Autodesk Fusion 360 part; units mm, degrees
sketch "Sketch1" plane through (0, 0, 0) normal (0, 1, 0) x (1, 0, 0)
  line L0 (13, 29) -> (-13, 29) construction
  line L1 (-13, 29) -> (-13, -29) construction
  line L2 (-13, -29) -> (13, -29) construction
  line L3 (13, -29) -> (13, 29) construction
  line L4 (13, 29) -> (-13, -29) construction
  line L5 (-13, 29) -> (13, -29) construction
  line L6 (0, 0) -> (0, 16.0365) construction
  line L7 (0, 0) -> (-11.1519, 0) construction
  line L8 (20, 36) -> (-20, 36)
  line L9 (-20, 36) -> (-20, -36)
  line L10 (-20, -36) -> (20, -36)
  line L11 (20, -36) -> (20, 36)
  line L12 (20, 36) -> (-20, -36) construction
  line L13 (-20, 36) -> (20, -36) construction
  circle A0 centre (13, 29) radius 1.75
  circle A1 centre (-13, 29) radius 1.75
  circle A2 centre (13, -29) radius 1.75
  circle A3 centre (-13, -29) radius 1.75
  line L14 (7.5, 36) -> (-7.5, 36)
  line L15 (-7.5, 36) -> (-7.5, 56)
  line L16 (-7.5, 56) -> (7.5, 56)
  line L17 (7.5, 56) -> (7.5, 36)
  line L18 (7.5, 36) -> (-7.5, 56) construction
  line L19 (-7.5, 36) -> (7.5, 56) construction
  circle A4 centre (0, 48) radius 3.4
  line L20 (7.5, -56) -> (7.5, -36)
  line L21 (-7.5, -56) -> (7.5, -56)
  line L22 (-7.5, -36) -> (-7.5, -56)
  circle A5 centre (0, -48) radius 3.4
  line L23 (7.5, -36) -> (-7.5, -36)
  point P0 (0, 46)
  dimension "d1" = 3.5
  dimension "d2" = 58
  dimension "d3" = 26
  dimension "d4" = 7
  dimension "d5" = 7
  dimension "d6" = 15
  dimension "d7" = 20
  dimension "d8" = 6.8
  dimension "d9" = 12
extrude "Extrude1" add sketch "Sketch1" along normal blind 4
fillet "Fillet1" radius 3 12 edges at (7.5, 2, 36) (20, 2, 36) (7.5, 2, 56) (-7.5, 2, 56) (-20, 2, 36) (-7.5, 2, 36) (20, 2, -36) (7.5, 2, -36) (7.5, 2, -56) (-7.5, 2, -56) (-20, 2, -36) (-7.5, 2, -36)
chamfer "Chamfer1" distance 2 angle 45 4 edges at (-14.6316, 4, -29.6328) (11.3684, 4, -29.6328) (11.3684, 4, 28.3672) (-14.6316, 4, 28.3672)
Can you work these out from the model? Positions are in its coordinate system, mm. A direction names the side the tool comes from. Coordinates: 2 decimals unless noted, no trailing zeros. Loops run counter-clockwise (first coordinate to the right, second up) from the corner with the lowest first, then second, coordinate; pieces in that order, holes last. Notation, with made-up numbers: M -29,89 L -17,89 A23 cw -17,116 Z; hole C 55,29 d1. An arc over 180 degrees is marked long. Return JSON: item names as keys, results as strings. Group by question number.
Item 1: If I drill on L1, parallel to X at y = 1.1, z = 29; L2, parallel to Z at x = -13, y = 2; L3, parallel to Z at x = 0, y = 2.8, over which ranges is the centre line in solid material (lowest first)? Write a range as from..to.
Item 2: Thinking about a two-plate mould opening in Z: for faces 1 (the cylindrical face through (-6.6, 2.03, -55.14)), 2 (the cylindrical face through (-19.14, 2.03, 35.1)), 3 (the cylindrical face through (13.81, 0.99, -30.55)), which applies, released by +Z, released by -Z, zero draft, split by the parting line, or undercut?
Item 3: Imagine slicing it at C-C (y = 2.7). Give the number of separate pieces and of enclosed holes in the cut face, and give its area (3 significant figures).
Item 4: On a 3-axis mill with a long thin cutter (end or side, diameter ignored), from which of +Z, -Z, +X, -X, +Y, -Y can I reach the whole of each face in a straight line? I mean faces 4 (the cylindrical face through (19.1, 2.03, 35.14)), 5 (the flat face through (0, 2, 56)), 6 (the flat face through (-7.5, 2, 46)), 7 (the flat face through (14, 2, -36)), 8 (the flat face through (-14, 2, -36)). Say none if no direction works.
Item 5: Imagine slicing it at B-B (z = -48). Please give me the cut outline in (x, y), and give its area (3 significant figures).
Item 6: I'm going to push flat-ended pins straight in: pin 1 Ø2 at (x, y) = (15.5, 0.5) entering from -Z; pin 2 Ø3 at (x, z) = (-13, 29) entering from +Y; pin 3 Ø10 at (x, z) = (10.5, 18.5) entering from -Y; pin 4 Ø2 at (y, z) = (2, -47.5) entering from -X. Where does each tip first touch, or does it pass through?
Item 7: Imagine slicing it at A-A (x = 13). Please give me the cut outline in (y, z), and give its area (3 significant figures).
Item 8: Imagine slicing it at D-D (z = 29). Please give me the cut outline in (x, y), and give its area (3 significant figures).
Verdict:
{
 "1": {"L1": "x = -20..-14.75, -11.25..11.25, 14.75..20", "L2": "z = -36..-30.75, -27.25..27.25, 30.75..36", "L3": "z = -56..-51.4, -44.6..44.6, 51.4..56"},
 "2": {"face 1": "released by -Z", "face 2": "released by +Z", "face 3": "undercut"},
 "3": {"separate pieces": "1", "enclosed holes": "6", "area": "3,320 mm^2"},
 "4": {"face 4": "+Z, +X, +Y, -Y", "face 5": "+Z, +X, -X, +Y, -Y", "face 6": "+Z, -X, +Y, -Y", "face 7": "-Z, +X, +Y, -Y", "face 8": "-Z, -X, +Y, -Y"},
 "5": {"outline": "M -7.5,0 L -3.4,0 L -3.4,4 L -7.5,4 Z; M 3.4,0 L 7.5,0 L 7.5,4 L 3.4,4 Z", "area": "32.8 mm^2"},
 "6": {"pin 1": "stops at z = -36", "pin 2": "passes through", "pin 3": "stops at y = 0", "pin 4": "stops at x = -7.5"},
 "7": {"outline": "M 0,-36 L 4,-36 L 4,-32.75 L 2,-30.75 L 0,-30.75 Z; M 0,-27.25 L 2,-27.25 L 4,-25.25 L 4,25.25 L 2,27.25 L 0,27.25 Z; M 0,30.75 L 2,30.75 L 4,32.75 L 4,36 L 0,36 Z", "area": "252 mm^2"},
 "8": {"outline": "M -20,0 L -14.75,0 L -14.75,2 L -16.75,4 L -20,4 Z; M -11.25,0 L 11.25,0 L 11.25,2 L 9.25,4 L -9.25,4 L -11.25,2 Z; M 14.75,0 L 20,0 L 20,4 L 16.75,4 L 14.75,2 Z", "area": "124 mm^2"}
}
